Design review of the part built by this model. Coordinates are the model's own, in mm. Face numbers are marked on the shaded views. A direction names the side the tool comes from. Coordinates: 2 decimals unless noted, no trailing zeros. Order: outer loops, then holes, each group sorted by start corner. A loop starts at its lowest first (then second) coordinate and runs counter-clockwise, first axis right, second up. Notation, with made-up numbers: (41.25, 49.25) -> (77.25, 49.25) arc R15 cw to (77.25, 72.25) -> close; hole circle Ø5 at (-2, -1.5). An arc over 180 degrees is marked (long way). Write item = value, one per line.
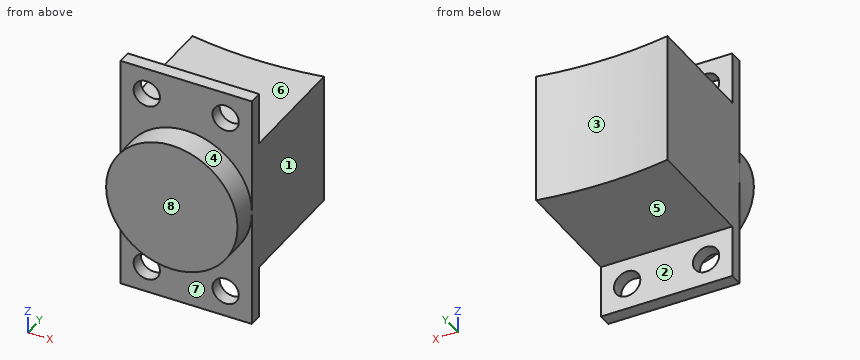
```python
from build123d import *

# Parameters (mm, degrees)
BOSS_EXTRUDE1_DEPTH      = 50
SKETCH2_R                = 25
BOSS_EXTRUDE2_DEPTH      = 10
BOSS_EXTRUDE3_DEPTH      = 20
BOSS_EXTRUDE3_DEPTH_BACK = 70
SKETCH3_W                = 50
SKETCH3_H                = 5
SKETCH4_R                = 5
CUT_EXTRUDE1_DEPTH       = 10


with BuildPart() as part:
    # Sketch1 → Boss-Extrude1 (new body)
    with BuildSketch(Plane.XY):
        with BuildLine():
            Line((25, 25), (25, -25))
            Line((25, -25), (-25, -25))
            Line((-25, -25), (-25, 25))
            ThreePointArc((-25, 25), (0, 22.791003179), (25, 25))
        make_face()
    extrude(amount=BOSS_EXTRUDE1_DEPTH)

    # Sketch2 → Boss-Extrude2 (add)
    with BuildSketch(Plane.XZ.offset(25)):
        with Locations((0, 25)):
            Circle(SKETCH2_R)
    extrude(amount=BOSS_EXTRUDE2_DEPTH)

    # Sketch3 → Boss-Extrude3 (add, two sides: drawn at the far end of the back side and taken through both)
    with BuildSketch(Plane.XY.offset(50).offset(-BOSS_EXTRUDE3_DEPTH_BACK)):
        with Locations((0, -22.5)):
            Rectangle(SKETCH3_W, SKETCH3_H)
    extrude(amount=BOSS_EXTRUDE3_DEPTH + BOSS_EXTRUDE3_DEPTH_BACK)

    # Sketch4 → Cut-Extrude1 (cut)
    with BuildSketch(Plane(origin=(0, -20, 0), x_dir=(1, 0, 0), z_dir=(0, 1, 0))):
        with Locations(Location((-15, -60, 0), (0, 0, 270))):
            Circle(SKETCH4_R)
        with Locations(Location((15, -60, 0), (0, 0, 270))):
            Circle(SKETCH4_R)
        with Locations(Location((15, 10, 0), (0, 0, 270))):
            Circle(SKETCH4_R)
        with Locations(Location((-15, 10, 0), (0, 0, 270))):
            Circle(SKETCH4_R)
    extrude(amount=-CUT_EXTRUDE1_DEPTH, mode=Mode.SUBTRACT)


solid = part.part
```
(1) We need section B-B (y = -21). Write out the cut boundary in (x, z).
Report:
outline = (-25, -20) -> (25, -20) -> (25, 70) -> (-25, 70) -> close; hole circle Ø10 at (-15, -10); hole circle Ø10 at (-15, 60); hole circle Ø10 at (15, -10); hole circle Ø10 at (15, 60)
(2) For the marked faces 4, 5, 6, 7 and 8, list the 3-axis set-ups (+Z, -Z, +X, -X, +Y, -Y) from which the entire face can be reached by the end or side of a thin tool; tool diameter is ignored.
Report:
face_4 = -Y
face_5 = -Z, +X, -X, +Y
face_6 = +Z, +X, -X, +Y
face_7 = -Z, -Y
face_8 = +Z, -Z, +X, -X, -Y
(3) The part is to be moulded in two halves that separate along X. For the marked faces 1, 2 and 3, say which applies: released by +X, released by -X, zero draft, split by the parting line, or undercut.
Report:
face_1 = released by +X
face_2 = zero draft
face_3 = undercut
(4) We need section C-C (x = 0). Write out the cut boundary in (y, z).
Report:
outline = (-35, 0) -> (-25, 0) -> (-25, -20) -> (-20, -20) -> (-20, 0) -> (22.79, 0) -> (22.79, 50) -> (-20, 50) -> (-20, 70) -> (-25, 70) -> (-25, 50) -> (-35, 50) -> close
(5) For L1, parallel to X at y = -21, z = -10; L2, parallel to Z at x = 10, y = -12; L3, parallel to Y at x = -15, z = 50.5, list the stretches that pass through material, from the lowest coordinate up.
Report:
L1 = -25 to -20, -10 to 10, 20 to 25
L2 = 0 to 50
L3 = -25 to -20
(6) We need section D-D (z = 29). Write out the cut boundary in (x, y), and give its area (3 significant figures).
Report:
outline = (-25, -25) -> (-24.68, -25) -> (-24.68, -35) -> (24.68, -35) -> (24.68, -25) -> (25, -25) -> (25, 25) arc R142.57 cw to (-25, 25) -> close
area = 2,920 mm²
(7) We need section A-A (z = -10). Write out the cut boundary in (x, y).
Report:
outline = (-25, -25) -> (-20, -25) -> (-20, -20) -> (-25, -20) -> close; (-10, -25) -> (10, -25) -> (10, -20) -> (-10, -20) -> close; (20, -25) -> (25, -25) -> (25, -20) -> (20, -20) -> close
(8) Insertion check: pin 1 (22 mm diameter, centred on x = 11, z = 58.5, fed in from +Y); pin 2 (11.5 mm diameter, centred on x = 15, z = -10, fed in from +Y); pin 3 (1 mm diameter, centred on x = -16, y = -26, fed in from -Z); pin 4 (8 mm diameter, centred on x = -15, z = -10, fed in from +Y). Each pin has a flat end and moves straight along its axis. Give the tip position at first contact, or say it passes through.
Report:
pin_1 = 23.93
pin_2 = -20
pin_3 = 5.38
pin_4 = through
